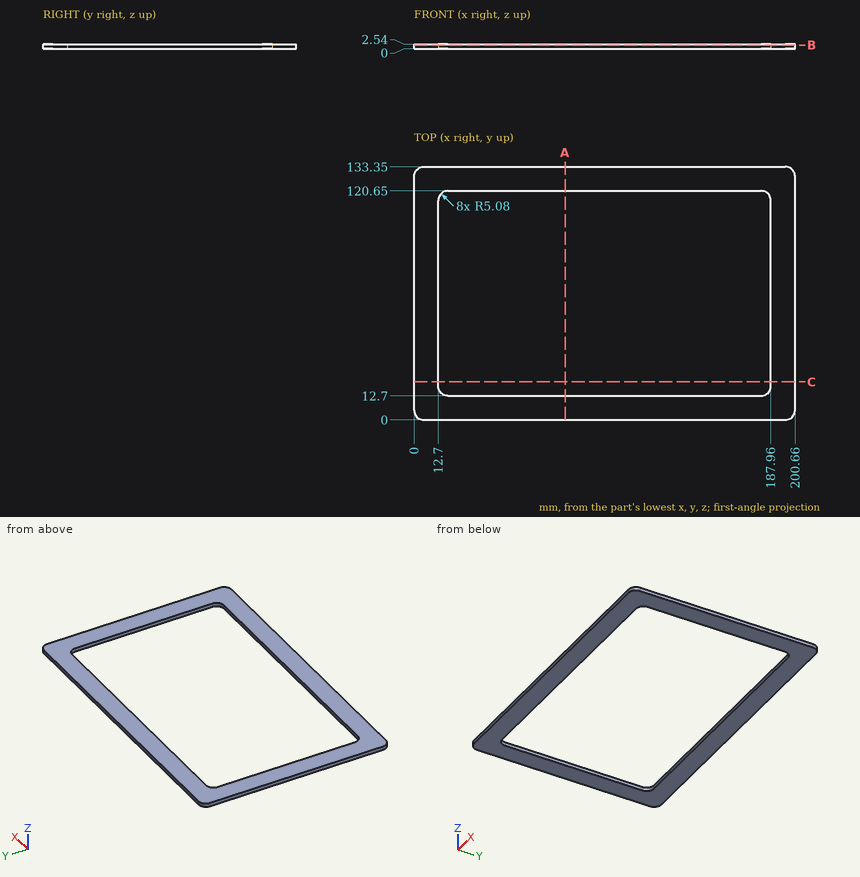
For this review, use the dimensioned drawing (mm, ordinates from the lowest corner) and the shaded views. Give positions to 0.01 mm unless a question says otherwise; leave off trailing zeros. Order: outer loops, then holes, each group sorted by start corner. A loop starts at its lowest first (then second) coordinate and runs counter-clockwise, first axis right, second up.
1) Take a section at C-C (y = 20). Give the boundary of the cut face in (x, z).
2) Insertion check: pin 1 (1.3 mm diameter, centred on y = 55, z = 1, fed in from -X). The pin has a flat end and moves straight along its axis. Give the tip position at first contact, or say it passes through.
3) Wall thickness on line 1 (X direction, y = 56, z = 1.5); line 2 (Y direction, x = 47, z = 1.7); line 3 (X direction, y = 119, z = 1.3): over which ranges is each line inside the solid? List them lowest first.
4) Take a section at B-B (z = 1.95). Give the boundary of the cut face in (x, y), then the cut area to 3 significant figures.
5) Take a section at A-A (x = 79.5). Give the boundary of the cut face in (y, z).
Derived:
1. outline: (0, 0) - (12.7, 0) - (12.7, 2.54) - (0, 2.54) - close; (187.96, 0) - (200.66, 0) - (200.66, 2.54) - (187.96, 2.54) - close
2. pin 1: stops at x = 0
3. line 1: x = 0 to 12.7, 187.96 to 200.66
3. line 2: y = 0 to 12.7, 120.65 to 133.35
3. line 3: x = 0 to 14.03, 186.63 to 200.66
4. outline: (0, 5.08) arc R5.08 ccw to (5.08, 0) - (195.58, 0) arc R5.08 ccw to (200.66, 5.08) - (200.66, 128.27) arc R5.08 ccw to (195.58, 133.35) - (5.08, 133.35) arc R5.08 ccw to (0, 128.27) - close; hole (12.7, 17.78) arc R5.08 ccw to (17.78, 12.7) - (182.88, 12.7) arc R5.08 ccw to (187.96, 17.78) - (187.96, 115.57) arc R5.08 ccw to (182.88, 120.65) - (17.78, 120.65) arc R5.08 ccw to (12.7, 115.57) - close
4. area: 7,840 mm2
5. outline: (0, 0) - (12.7, 0) - (12.7, 2.54) - (0, 2.54) - close; (120.65, 0) - (133.35, 0) - (133.35, 2.54) - (120.65, 2.54) - close
